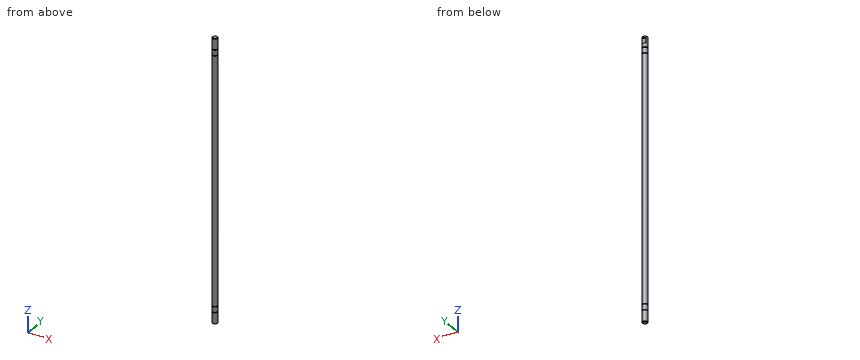
from build123d import *

# Parameters (mm, degrees)
SKETCH1_R           = 3
BOSS_EXTRUDE1_DEPTH = 330
CUT_EXTRUDE1_START  = -13
SKETCH2_R           = 3
SKETCH2_R_2         = 2.85
CUT_EXTRUDE1_DEPTH  = 0.8
CUT_EXTRUDE2_START  = -6
SKETCH3_R           = 3
SKETCH3_R_2         = 2.85
CUT_EXTRUDE2_DEPTH  = 0.8
CUT_EXTRUDE3_START  = -296
SKETCH3_2_R         = 3
SKETCH3_2_R_2       = 2.85
CUT_EXTRUDE3_DEPTH  = 0.8
CUT_EXTRUDE4_START  = -302.8
SKETCH3_3_R         = 3
SKETCH3_3_R_2       = 2.85
CUT_EXTRUDE4_DEPTH  = 0.8
CUT_EXTRUDE5_START  = 3
SKETCH4_W           = 6
SKETCH4_H           = 6
CUT_EXTRUDE5_DEPTH  = 1
CHAMFER1_SIZE       = 0.5


with BuildPart() as part:
    # Sketch1 → Boss-Extrude1 (new body)
    with BuildSketch(Plane.XY):
        Circle(SKETCH1_R)
    extrude(amount=BOSS_EXTRUDE1_DEPTH)

    # Sketch2 → Cut-Extrude1 (cut)
    with BuildSketch(Plane(origin=(0, 0, 0), x_dir=(-1, 0, 0), z_dir=(0, 0, -1)).offset(CUT_EXTRUDE1_START)):
        Circle(SKETCH2_R)
        Circle(SKETCH2_R_2, mode=Mode.SUBTRACT)
    extrude(amount=-CUT_EXTRUDE1_DEPTH, mode=Mode.SUBTRACT)

    # Sketch3 → Cut-Extrude2 (cut)
    with BuildSketch(Plane(origin=(0, 0, 13.8), x_dir=(-1, 0, 0), z_dir=(0, 0, -1)).offset(CUT_EXTRUDE2_START)):
        Circle(SKETCH3_R)
        Circle(SKETCH3_R_2, mode=Mode.SUBTRACT)
    extrude(amount=-CUT_EXTRUDE2_DEPTH, mode=Mode.SUBTRACT)

    # Sketch3<2> → Cut-Extrude3 (cut)
    with BuildSketch(Plane(origin=(0, 0, 13.8), x_dir=(-1, 0, 0), z_dir=(0, 0, -1)).offset(CUT_EXTRUDE3_START)):
        Circle(SKETCH3_2_R)
        Circle(SKETCH3_2_R_2, mode=Mode.SUBTRACT)
    extrude(amount=-CUT_EXTRUDE3_DEPTH, mode=Mode.SUBTRACT)

    # Sketch3<3> → Cut-Extrude4 (cut)
    with BuildSketch(Plane(origin=(0, 0, 13.8), x_dir=(-1, 0, 0), z_dir=(0, 0, -1)).offset(CUT_EXTRUDE4_START)):
        Circle(SKETCH3_3_R)
        Circle(SKETCH3_3_R_2, mode=Mode.SUBTRACT)
    extrude(amount=-CUT_EXTRUDE4_DEPTH, mode=Mode.SUBTRACT)

    # Sketch4 → Cut-Extrude5 (cut)
    with BuildSketch(Plane(origin=(0, 0, 0), x_dir=(1, 0, 0), z_dir=(0, 1, 0)).offset(CUT_EXTRUDE5_START)):
        with Locations((0, -324.9)):
            Rectangle(SKETCH4_W, SKETCH4_H)
    extrude(amount=-CUT_EXTRUDE5_DEPTH, mode=Mode.SUBTRACT)

    # Chamfer1
    chamfer1_edges = [part.edges().sort_by_distance(p)[0] for p in [
        (-3, 0, 0),
        (-3, 0, 330),
    ]]
    chamfer(chamfer1_edges, length=CHAMFER1_SIZE)


solid = part.part
Geometry: final body of the model. Coordinates: model frame, mm. Give positions to 0.01 mm unless a question says otherwise; leave off trailing zeros. Order: outer loops, then holes, each group sorted by start corner. A loop starts at its lowest first (then second) coordinate and runs counter-clockwise, first axis right, second up. Notation, with made-up numbers: (12.25, -20.5) -> (67.25, -20.5) arc R30 cw to (67.25, 17.5) -> close; hole circle Ø3 at (-32, 14.25). An arc over 180 degrees is marked (long way). Answer as a JSON object with one key per item and string values.
Q1. Section A-A (z = 288). Output: boundary loops of the cut face in (x, y).
Entries:
{"outline": "circle Ø6 at (0, 0)"}
Q2. First-contact query: pin 1 (1 mm diameter, centred on y = 1.5, z = 158.5, fed in from +X); pin 2 (2 mm diameter, centred on x = -0.5, z = 324, fed in from +Y). Flat tips, straight axial feed; report the tip coordinate or a pass-through.
Entries:
{"pin 1": "stops at x = 2.83", "pin 2": "stops at y = 2"}
Q3. Material intervals for probe 1 along Z at (x, y) = (1, 2.05); probe 2 along Y at (x, z) = (1.6, 313.5); probe 3 along Z at (x, y) = (1.8, 2.25), sorted ascending.
Entries:
{"probe 1": "z = 0 to 321.9, 327.9 to 330", "probe 2": "y = -2.54 to 2.54", "probe 3": "z = 0.38 to 13, 13.8 to 19.8, 20.6 to 309.8, 310.6 to 316.6, 317.4 to 321.9, 327.9 to 329.62"}
